```python
from build123d import *

# Parameters (mm, degrees)
F0_W        = 5
F0_H        = 2.5
F0_H_2      = 23.5
F0_H_3      = 4
F1_DEPTH    = 5
F2_W        = 5.5
F2_H        = 5.6794419712
F3_DEPTH    = 6.5
F4_R        = 1.75
F5_DEPTH    = 25.4
F6_W        = 5
F6_H        = 24.5096784085
F6_W_2      = 23
F6_H_2      = 5
F7_DEPTH    = 2
F8_T1_DEPTH = 5
F9_W        = 6.5
F9_H        = 5
F10_DEPTH   = 2
F11_R       = 2.5
F12_DEPTH   = 36.501


# Not quite as in the source:
# - a fillet or chamfer that OpenCascade refuses, or shapes differently, is made with other operations: its cross-section is extruded or revolved along the edge and cut away or added


with BuildPart() as f1:
    # F0 (on Front) → F1 (new body)
    with BuildSketch(Plane.XZ):
        with Locations((0, 13.75)):
            Rectangle(F0_W, F0_H)
        Polygon((-2.5, 15), (2.5, 15), (2.5, 12.5), (25.5, 12.5), (25.5, 17.5), (-25.5, 17.5), (-25.5, 12.5), (-2.5, 12.5), align=None)
        with Locations((0, 0.75)):
            Rectangle(F0_W, F0_H_2)
        Polygon((7.5, -11), (2.5, -11), (2.5, -15), (-2.5, -15), (-2.5, -11), (-7.5, -11), (-7.5, -19), (7.5, -19), align=None)
        with Locations((0, -13)):
            Rectangle(F0_W, F0_H_3)
    extrude(amount=F1_DEPTH)

    # F2 (on face) → F3 (cut)
    with BuildSketch(Plane(origin=(0, 0, -19), x_dir=(1, 0, 0), z_dir=(0, 0, -1))):
        with Locations((0, 2.1602790144)):
            Rectangle(F2_W, F2_H)
    extrude(amount=-F3_DEPTH, mode=Mode.SUBTRACT)

    # F4 (on face) → F5 (cut)
    with BuildSketch(Plane(origin=(-7.5, 0, 0), x_dir=(0, -1, 0), z_dir=(-1, 0, 0))):
        with Locations((2.5, -15)):
            Circle(F4_R)
    extrude(amount=-F5_DEPTH, mode=Mode.SUBTRACT)

    # F6 (on face) → F7 (cut)
    with BuildSketch(Plane.XZ.offset(5)):
        with Locations((0, 0.2451607957)):
            Rectangle(F6_W, F6_H)
        with Locations((-14, 15)):
            Rectangle(F6_W_2, F6_H_2)
        with Locations((0, 15)):
            Rectangle(F6_W, F6_H_2)
        with Locations((14, 15)):
            Rectangle(F6_W_2, F6_H_2)
    extrude(amount=-F7_DEPTH, mode=Mode.SUBTRACT)

    # F8: fillet of radius 5.08 on 1 edges, made by hand

    # F8_s2 → F8_t1 (join)
    with BuildSketch(Plane.YZ.offset(-2.5)):
        with BuildLine():
            ThreePointArc((-3, -7.9698764332), (-3.5273743839, -10.2237619671), (-5, -12.0096784085))
            Line((-5, -12.0096784085), (-3, -12.0096784085))
            Line((-3, -12.0096784085), (-3, -7.9698764332))
        make_face()
    extrude(amount=F8_T1_DEPTH)

    # F9 (on face) → F10 (join)
    with BuildSketch(Plane.XZ.offset(3)):
        with Locations((22.25, 15)):
            Rectangle(F9_W, F9_H)
        with Locations((-22.25, 15)):
            Rectangle(F9_W, F9_H)
    extrude(amount=F10_DEPTH)

    # F11 (on face) → F12 (cut, through all)
    with BuildSketch(Plane.XY.offset(17.5)):
        with Locations((22.25, -5)):
            Circle(F11_R)
        with Locations((-22.25, -5)):
            Circle(F11_R)
    extrude(amount=-F12_DEPTH, mode=Mode.SUBTRACT)


solid = f1.part
```
The listing builds one solid part. Answer for the finished solid, in the listing's coordinates (mm). A direction names the side the tool comes from. Round coordinates to 2 decimals unless told otherwise and drop trailing zeros. Loops run counter-clockwise (first coordinate to the right, second up) from the corner with the lowest first, then second, coordinate; pieces in that order, holes last.
1) A cutting plane is placed at C-C on x = 22.25. Determine the outline of the cut face in (y, z), plus the area to 3 significant figures.
Outcome:
outline: (-2.5, 12.5) - (0, 12.5) - (0, 17.5) - (-2.5, 17.5) - close
area: 12.5 mm2
2) Given P1, Ø2.5, axis at y = -1.5, z = -13.5, coming from the -X side; P2, Ø1.5, axis at x = 0, y = -3, coming from the -Z side; P3, Ø3, axis at y = -3, z = -1.5, coming from the +X side; P4, Ø1.5, axis at x = 6, y = -3.5, coming from the +Z side, each flat-ended and moving along its own axis, determine where each tip first touches the part or whether it passes through.
Outcome:
P1: stops at x = -7.5
P2: stops at z = -12.5
P3: stops at x = 2.5
P4: stops at z = 17.5
3) For a pull along Y with two mould halves and no side action, classify faces 5 (the face through (-2.75, -2, -17)), 6 (the face through (5.092, -2.272, -13.265)), 7 (the face through (-22.2, -2.5, 15)) as released by +Y, released by -Y, zero draft, split by the parting line, or undercut.
Outcome:
face 5: zero draft
face 6: undercut
face 7: released by -Y
4) For faces 1 (the face through (0, -3, -12.5)), 2 (the face through (14, -1, 12.5)), 3 (the face through (-14, -1, 12.5)), 4 (the face through (0, -3, 11)), determine the directions among +Z, -Z, +X, -X, +Y, -Y from which every point of the face is accessible in a straight line to the end or side of a thin tool.
Outcome:
face 1: -Z, +Y, -Y
face 2: +X, +Y, -Y
face 3: -X, +Y, -Y
face 4: +Z, -Y
5) Consider line 1 (Z direction, x = -5.8, y = -2.5); line 2 (Y direction, x = -7, z = 16.5); line 3 (Z direction, x = 5.5, y = -4.1). Determine where each line is inside the solid, lowest interval first.
Outcome:
line 1: z = -19 to -16.75, -13.25 to -11, 12.5 to 17.5
line 2: y = -3 to 0
line 3: z = -19 to -15.71, -14.29 to -11
6) A cutting plane is placed at A-A on x = 6. Determine the outline of the cut face in (y, z), plus the area to 3 significant figures.
Outcome:
outline: (-5, -19) - (0, -19) - (0, -11) - (-5, -11) - close; (-3, 12.5) - (0, 12.5) - (0, 17.5) - (-3, 17.5) - close; hole circle Ø3.5 at (-2.5, -15)
area: 45.4 mm2
7) A cutting plane is placed at B-B on z = -15. Determine the outline of the cut face in (x, y).
Outcome:
outline: (-7.5, -5) - (-2.75, -5) - (-2.75, -4.25) - (-7.5, -4.25) - close; (-7.5, -0.75) - (-2.75, -0.75) - (-2.75, 0) - (-7.5, 0) - close; (2.75, -5) - (7.5, -5) - (7.5, -4.25) - (2.75, -4.25) - close; (2.75, -0.75) - (7.5, -0.75) - (7.5, 0) - (2.75, 0) - close
8) A cutting plane is placed at D-D on z = 1. Determine the outline of the cut face in (x, y), plus the area to 3 significant figures.
Outcome:
outline: (-2.5, -3) - (2.5, -3) - (2.5, 0) - (-2.5, 0) - close
area: 15.0 mm2
